```python
from build123d import *

# Parameters (mm, degrees)
M6_CLEARANCE_HOLE1_D = 6.6
SKETCH6_R            = 5.25
CUT_EXTRUDE1_DEPTH   = 7.5
FILLET1_R            = 0.5


with BuildPart() as part:
    # Sketch2 → Revolve1 (revolve)
    with BuildSketch(Plane.XY):
        with BuildLine():
            Line((0, 0), (12.7, 0))
            ThreePointArc((12.7, 0), (8.980256121, 8.980256121), (0, 12.7))
            Line((0, 12.7), (0, 0))
        make_face()
    revolve(axis=Axis((0, 0, 0), (0, 1, 0)))

    # M6 Clearance Hole1 (through all)
    with Locations(Plane(origin=(0, 0, 0), x_dir=(-1, 0, 0), z_dir=(0, -1, 0))):
        with Locations((0, 0)):
            Hole(M6_CLEARANCE_HOLE1_D / 2)

    # Sketch6 → Cut-Extrude1 (cut)
    with BuildSketch(Plane(origin=(0, 12.263767773, 0), x_dir=(1, 0, 0), z_dir=(0, 1, 0))):
        with Locations(Location((0, 0, 0), (0, 0, 270))):
            Circle(SKETCH6_R)
    extrude(amount=-CUT_EXTRUDE1_DEPTH, mode=Mode.SUBTRACT)

    # Fillet1
    fillet1_edges = [part.edges().sort_by_distance(p)[0] for p in [
        (-3.712310601, 11.564060705, -3.712310601),
    ]]
    fillet(fillet1_edges, radius=FILLET1_R)


solid = part.part
```
Verification items for the finished model (mm, model axes). A direction names the side the tool comes from. Give positions to 0.01 mm unless a question says otherwise; leave off trailing zeros. Order: outer loops, then holes, each group sorted by start corner. A loop starts at its lowest first (then second) coordinate and runs counter-clockwise, first axis right, second up. Notation, with made-up numbers: M 76,41.5 L 134,41.5 A25 cw 134,63.5 Z; hole C 73.25,33.5 d6. An arc over 180 degrees is marked long. Answer in a Markdown table with one row per item. Add a question column.
Item 1: Scan lines: probe 1 along X at (y, z) = (8.5, 4); probe 2 along Y at (x, z) = (-5.5, -0.5); probe 3 along X at (y, z) = (1.5, 0.5). Record each from-to range of solid material in increasing order. Write a range as from..to.
Item 2: Gauge pin test, flat ends, axial feed: pin 1 (3 mm diameter, centred on y = 6.5, z = 0, fed in from +X); pin 2 (3 mm diameter, centred on y = 1.5, z = -3, fed in from +X); pin 3 (3 mm diameter, centred on x = 2, z = -2.5, fed in from +Y); pin 4 (5.5 mm diameter, centred on x = 0, z = 0, fed in from +Y). Record the tip position at first contact, or that the pin passes through.
Item 3: Section check B-B, the plane x = -9. Enter the section's corners in (y, z).
Item 4: Tool access check on faces 1 (the cylindrical face through (-2.43, 2.42, -2.23)), 2 (the cylindrical face through (1.6, 7.8, 5)). Record the directions out of +Z, -Z, +X, -X, +Y, -Y that give a thin tool (end or side, any length) a straight path to the whole face; none if there is none.
Item 5: Section check C-C, the plane z = -8.75. Enter the section's corners in (x, y).
Item 6: Section check D-D, the plane y = 8.25. Enter the section's corners in (x, z).
Item 7: Mould release check, pull along X, two halves, no side actions. Record for faces 3 (the flat face through (-1.1, 4.764, 3.4)), 4 (the flat face through (-3, 0, 3)): released by +X, released by -X, zero draft, split by the parting line, or undercut.
Filled sheet:
| question | item | result |
|---|---|---|
| 1 | probe 1 | x = -8.55..-3.4, 3.4..8.55 |
| 1 | probe 2 | y = 0..11.21 |
| 1 | probe 3 | x = -12.6..-3.26, 3.26..12.6 |
| 2 | pin 1 | stops at x = 11.67 |
| 2 | pin 2 | stops at x = 12.56 |
| 2 | pin 3 | stops at y = 4.76 |
| 2 | pin 4 | passes through |
| 3 | outline | M 0,-8.96 A8.96 ccw 0,8.96 Z |
| 4 | face 1 | +Y, -Y |
| 4 | face 2 | +Y |
| 5 | outline | M -9.2,0 L 9.2,0 A9.2 ccw Z |
| 6 | outline | C 0,0 d19.31; hole C 0,0 d10.5 |
| 7 | face 3 | undercut |
| 7 | face 4 | zero draft |
